Can you work these out from the model? Positions are in its coordinate system, mm. Face numbers are marked on the shaded views. Round coordinates to 2 decimals unless told otherwise and drop trailing zeros. Loops run counter-clockwise (first coordinate to the right, second up) from the corner with the lowest first, then second, coordinate; pieces in that order, holes last. Notation, with made-up numbers: M 10.5,55.25 L 19.5,55.25 A24 cw 19.5,89.25 Z; hole C -29,53 d1. An arc over 180 degrees is marked long. Answer as CSV lines item,"result".
from build123d import *

# Parameters (mm, degrees)
SKETCH1_R           = 31.75
BOSS_EXTRUDE1_DEPTH = 5.588
SKETCH2_R           = 2.0955
CUT_EXTRUDE1_DEPTH  = 7.62
SKETCH5_R           = 3.4544
CUT_EXTRUDE2_DEPTH  = 3.4544
SKETCH6_R           = 3.175
CUT_EXTRUDE3_DEPTH  = 46.247660094
SKETCH9_R           = 29.21
SKETCH9_R_2         = 26.67
BOSS_EXTRUDE3_DEPTH = 3.81


with BuildPart() as part:
    # Sketch1 → Boss-Extrude1 (new body)
    with BuildSketch(Plane(origin=(0, 0, 0), x_dir=(1, 0, 0), z_dir=(0, 1, 0))):
        with Locations(Location((0, 0, 0), (0, 0, 270))):
            Circle(SKETCH1_R)
    extrude(amount=-BOSS_EXTRUDE1_DEPTH)

    # Sketch2 → Cut-Extrude1 (cut)
    with BuildSketch(Plane.XZ.offset(5.588)):
        with Locations(Location((0, 13.97, 0), (0, 0, 270))):
            Circle(SKETCH2_R)
        with Locations(Location((12.098374891, 6.985, 0), (0, 0, 270))):
            Circle(SKETCH2_R)
        with Locations(Location((12.098374891, -6.985, 0), (0, 0, 270))):
            Circle(SKETCH2_R)
        with Locations(Location((0, -13.97, 0), (0, 0, 270))):
            Circle(SKETCH2_R)
        with Locations(Location((-12.098374891, -6.985, 0), (0, 0, 270))):
            Circle(SKETCH2_R)
        with Locations(Location((-12.098374891, 6.985, 0), (0, 0, 270))):
            Circle(SKETCH2_R)
    extrude(amount=-CUT_EXTRUDE1_DEPTH, mode=Mode.SUBTRACT)

    # Sketch5 → Cut-Extrude2 (cut)
    with BuildSketch(Plane(origin=(0, 0, 0), x_dir=(1, 0, 0), z_dir=(0, 1, 0))):
        with Locations(Location((12.098374891, -6.985, 0), (0, 0, 270))):
            Circle(SKETCH5_R)
        with Locations(Location((0, -13.97, 0), (0, 0, 270))):
            Circle(SKETCH5_R)
        with Locations(Location((-12.098374891, -6.985, 0), (0, 0, 270))):
            Circle(SKETCH5_R)
        with Locations(Location((-12.098374891, 6.985, 0), (0, 0, 270))):
            Circle(SKETCH5_R)
        with Locations(Location((0, 13.97, 0), (0, 0, 270))):
            Circle(SKETCH5_R)
        with Locations(Location((12.098374891, 6.985, 0), (0, 0, 270))):
            Circle(SKETCH5_R)
    extrude(amount=-CUT_EXTRUDE2_DEPTH, mode=Mode.SUBTRACT)

    # Sketch6 → Cut-Extrude3 (cut, through all)
    with BuildSketch(Plane.XZ.offset(5.588)):
        with Locations(Location((0, 0, 0), (0, 0, 270))):
            Circle(SKETCH6_R)
    extrude(amount=-CUT_EXTRUDE3_DEPTH, mode=Mode.SUBTRACT)

    # Sketch9 → Boss-Extrude3 (add)
    with BuildSketch(Plane(origin=(0, 0, 0), x_dir=(1, 0, 0), z_dir=(0, 1, 0))):
        with Locations(Location((0, 0, 0), (0, 0, 90))):
            Circle(SKETCH9_R)
        with Locations(Location((0, 0, 0), (0, 0, 90))):
            Circle(SKETCH9_R_2, mode=Mode.SUBTRACT)
    extrude(amount=BOSS_EXTRUDE3_DEPTH)


solid = part.part
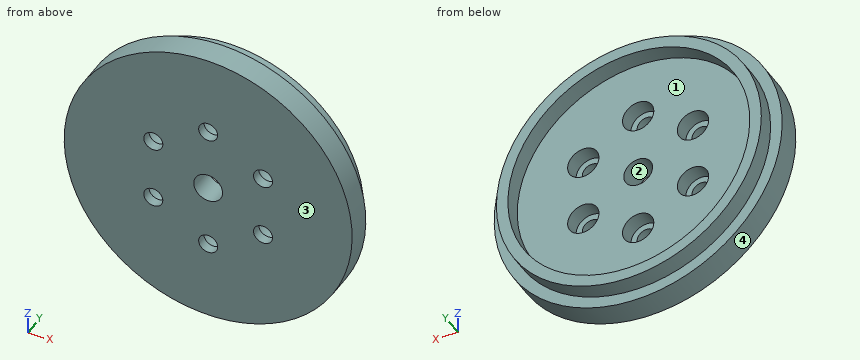
Item 1: Will these pins go through, and if not, where does the flat tip stop? pin 1 (2 mm diameter, centred on x = -11.5, z = 7, fed in from +Y); pin 2 (1 mm diameter, centred on y = 1, z = -19, fed in from +X); pin 3 (9 mm diameter, centred on x = -12.1, z = 6.98, fed in from +Y); pin 4 (2 mm diameter, centred on x = 1, z = 15, fed in from +Y).
Output:
pin 1,"passes through"
pin 2,"stops at x = 22.6"
pin 3,"stops at y = 0"
pin 4,"stops at y = -3.45"
Item 2: If I drill on line 1 along Z through (x, y) = (-11, -0.25); line 2 along X through (y, z) = (3, 14); line 3 along Z through (x, y) = (1, 3), over which ranges is the centre line in solid material (lowest first)? Write a range as from..to.
Output:
line 1,"z = -29.78..-10.26, -3.71..3.71, 10.26..29.78"
line 2,"x = -25.64..-22.7, 22.7..25.64"
line 3,"z = -29.19..-26.65, 26.65..29.19"
Item 3: If we section it at D-D on y = 2: Write out the boundary of the cut face in (x, z).
Output:
outline,"C 0,0 d58.42; hole C 0,0 d53.34"
Item 4: If we section it at B-B on x = 0: State how many separate pieces and enclosed holes the cut face has, then the cut area to 3 significant figures.
Output:
separate pieces,"4"
enclosed holes,"0"
area,"273 mm2"
Item 5: If we section it at A-A on z = 0: Write out the boundary of the cut face in (x, y) (3 decimals).
Output:
outline,"M -31.75,-5.588 L -3.175,-5.588 L -3.175,0 L -26.67,0 L -26.67,3.81 L -29.21,3.81 L -29.21,0 L -31.75,0 Z; M 3.175,-5.588 L 31.75,-5.588 L 31.75,0 L 29.21,0 L 29.21,3.81 L 26.67,3.81 L 26.67,0 L 3.175,0 Z"
Item 6: We'd pull the mould along X, two halves only. Please class the marked faces 1, 2, 3 and 4: released by +X, released by -X, zero draft, split by the parting line, or undercut.
Output:
face 1,"undercut"
face 2,"undercut"
face 3,"zero draft"
face 4,"split by the parting line"
Item 7: If we section it at C-C on y = -1.5: Write out the boundary of the cut face in (x, z) (3 decimals), then the cut area to 3 significant figures.
Output:
outline,"C 0,0 d63.5; hole C -12.098,-6.985 d6.909; hole C -12.098,6.985 d6.909; hole C 0,-13.97 d6.909; hole C 0,13.97 d6.909; hole C 0,0 d6.35; hole C 12.098,-6.985 d6.909; hole C 12.098,6.985 d6.909"
area,"2,910 mm2"
